The drawing under review shows one solid part. Ordinate dimensions are in mm from its lowest x, y, z. A direction names the side the tool comes from. Give positions to 0.01 mm unless a question says otherwise; leave off trailing zeros. Put each result on its own line as item: value. Start each with the question number.
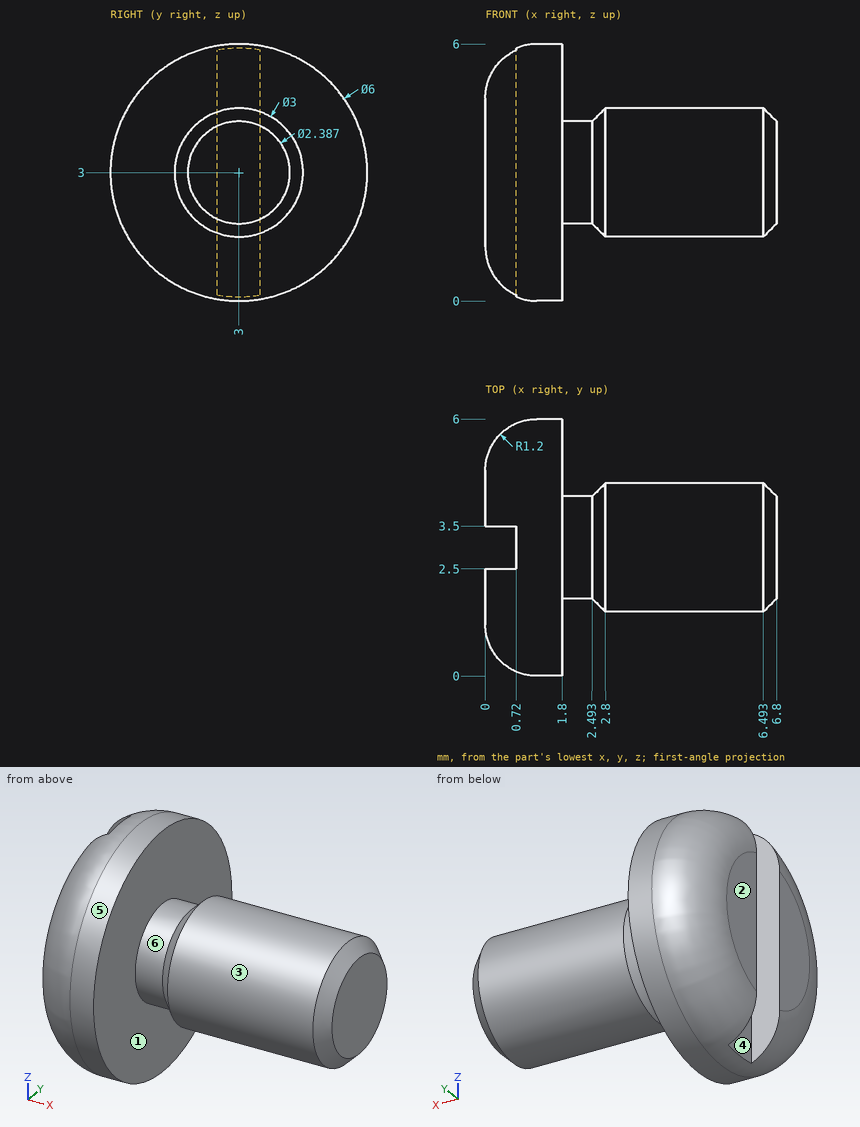
(1) Insertion check: pin 1 (0.8 mm diameter, centred on x = 0.5, z = 4, fed in from +Y); pin 2 (1 mm diameter, centred on x = 4.5, y = 2.5, fed in from +Z); pin 3 (0.8 mm diameter, centred on x = 0.5, z = 4, fed in from -Y). Each pin has a flat end and moves straight along its axis. Give the tip position at first contact, or say it passes through.
(2) Draft analysis for pull direction X (two halves, no side actions). For the marked faces 4, 5 and 6, state which applies: +X half, -X half, draft (parallel to the pull), parting line (faces both ways), or undercut.
(3) To check wall thickness, follow L1, parallel to Y at x = 0.5, z = 4; L2, parallel to Z at x = 3, y = 3; L3, parallel to X at y = 2.75, z = 1.75 (1 decimal). State the ranges of each line that lie inside material, in increasing order. Write a range as [from, to].
(4) For the marked faces 1, 2 and 3, list the 3-axis set-ups (+Z, -Z, +X, -X, +Y, -Y) from which the entire face can be reached by the end or side of a thin tool; tool diameter is ignored.
Check sheet entries:
1. pin 1: stops at y = 5.84
1. pin 2: stops at z = 4.5
1. pin 3: stops at y = 0.16
2. face 4: -X half
2. face 5: draft
2. face 6: undercut
3. L1: y = [0.41, 2.5], [3.5, 5.59]
3. L2: z = [1.5, 4.5]
3. L3: x = [0.7, 1.8], [2.6, 6.7]
4. face 1: none
4. face 2: +Z, -Z, -X, +Y, -Y
4. face 3: +X
